```python
from build123d import *

# Parameters (mm, degrees)
SKETCH1_R               = 2.413
BOSS_EXTRUDE1_DEPTH     = 1.7859375
SKETCH6_R               = 3.956130657
SKETCH6_R_2             = 2.413
BOSS_EXTRUDE2_DEPTH     = 0.381
SKETCH5_OUTSIDE_W       = 46.08
SKETCH5_OUTSIDE_H       = 47.552
SKETCH5_OUTSIDE_R       = 4.7625
CUT_EXTRUDE2_DEPTH      = 9.104416837
CUT_EXTRUDE2_DRAFT      = -60
MIRROR1_COPY_1_SKETCH_W = 46.08
MIRROR1_COPY_1_SKETCH_H = 47.552
MIRROR1_COPY_1_SKETCH_R = 4.7625
MIRROR1_COPY_1_DEPTH    = 9.104416837
MIRROR1_COPY_1_DRAFT    = -60


with BuildPart() as part:
    # Sketch1 → Boss-Extrude1 (new, symmetric)
    with BuildSketch(Plane(origin=(0, 0, 0), x_dir=(1, 0, 0), z_dir=(0, 1, 0))):
        Polygon((-4.7625, 2.749630657), (-4.7625, -2.749630657), (0, -5.499261314), (4.7625, -2.749630657), (4.7625, 2.749630657), (0, 5.499261314), align=None)
        with Locations(Location((0, 0, 0), (0, 0, 270))):
            Circle(SKETCH1_R, mode=Mode.SUBTRACT)
    extrude(amount=BOSS_EXTRUDE1_DEPTH, both=True)

    # Sketch6 → Boss-Extrude2 (add)
    with BuildSketch(Plane(origin=(0, 1.7859375, 0), x_dir=(1, 0, 0), z_dir=(0, 1, 0))):
        with Locations(Location((0, 0, 0), (0, 0, 90))):
            Circle(SKETCH6_R)
        with Locations(Location((0, 0, 0), (0, 0, 270))):
            Circle(SKETCH6_R_2, mode=Mode.SUBTRACT)
    extrude(amount=BOSS_EXTRUDE2_DEPTH)


with BuildPart() as cut_extrude2_tool:
    # Sketch5 outside → Cut-Extrude2 (with draft: the straight prism first)
    with BuildSketch(Plane(origin=(0, 1.7859375, 0), x_dir=(1, 0, 0), z_dir=(0, 1, 0))):
        Rectangle(SKETCH5_OUTSIDE_W, SKETCH5_OUTSIDE_H)
        Circle(SKETCH5_OUTSIDE_R, mode=Mode.SUBTRACT)
    extrude(amount=-CUT_EXTRUDE2_DEPTH)
    # Cut-Extrude2: the draft: its side faces are tilted about the plane it starts from
    cut_extrude2_sides = [cut_extrude2_tool.faces().sort_by_distance(p)[0] for p in [
        (0, -2.766270918, 23.776),
        (23.04, -2.766270918, 0),
        (0, -2.766270918, -23.776),
        (-23.04, -2.766270918, 0),
        (-4.7625, -2.766270918, 0),
    ]]
    draft(cut_extrude2_sides, Plane(origin=(0, 1.7859375, 0), x_dir=(1, 0, 0), z_dir=(0, 1, 0)), CUT_EXTRUDE2_DRAFT)


with BuildPart() as part_1:
    add(part.part)

    # Cut-Extrude2: cut by cut_extrude2_tool
    add(cut_extrude2_tool.part, mode=Mode.SUBTRACT)


with BuildPart() as mirror1_copy_1_tool:
    # Mirror1 copy 1 sketch → Mirror1 copy 1 (with draft: the straight prism first)
    with BuildSketch(Plane.XZ.offset(1.7859375)):
        Rectangle(MIRROR1_COPY_1_SKETCH_W, MIRROR1_COPY_1_SKETCH_H)
        Circle(MIRROR1_COPY_1_SKETCH_R, mode=Mode.SUBTRACT)
    extrude(amount=-MIRROR1_COPY_1_DEPTH)
    # Mirror1 copy 1: the draft: its side faces are tilted about the plane it starts from
    mirror1_copy_1_sides = [mirror1_copy_1_tool.faces().sort_by_distance(p)[0] for p in [
        (0, 2.766270918, 23.776),
        (23.04, 2.766270918, 0),
        (0, 2.766270918, -23.776),
        (-23.04, 2.766270918, 0),
        (-4.7625, 2.766270918, 0),
    ]]
    draft(mirror1_copy_1_sides, Plane.XZ.offset(1.7859375), MIRROR1_COPY_1_DRAFT)


with BuildPart() as part_2:
    add(part_1.part)

    # Mirror1 copy 1: cut by mirror1_copy_1_tool
    add(mirror1_copy_1_tool.part, mode=Mode.SUBTRACT)


solid = part_2.part
```
Work out the finished part from the listing and answer in its coordinate system (mm). A direction names the side the tool comes from. Give positions to 0.01 mm unless a question says otherwise; leave off trailing zeros. Order: outer loops, then holes, each group sorted by start corner. A loop starts at its lowest first (then second) coordinate and runs counter-clockwise, first axis right, second up. Notation, with made-up numbers: (-26, 72) - (-1, 72) arc R8 cw to (-1, 84) - close; hole circle Ø5 at (-19, -39). An arc over 180 degrees is marked (long way). One line per item, written item: value. Start each with the question number.
1. Section A-A, the plane y = -0.85 is taken. Write down the section's boundary in (x, z), then the cut area to 3 significant figures.
2. Each of these flat-tipped pins is pushed along its axis until it touches: pin 1 Ø1 at (x, z) = (3.5, -4) entering from -Y; pin 2 Ø1 at (y, z) = (-1, -4) entering from -X; pin 3 Ø2 at (x, y) = (2, -0.5) entering from -Z. Where does it stop, or does it pass through?
3. For a pull along X with two mould halves and no side action, classify faces 1 (the face through (-1.468, 0.163, -1.915)), 2 (the face through (4.762, 0, 0)), 3 (the face through (2, -1.786, 2)) as released by +X, released by -X, zero draft, split by the parting line, or undercut.
4. Which of the six approach directions +Z, -Z, +X, -X, +Y, -Y give full straight-line access (tool end or side, diameter ignored) to faces 4 (the face through (3.86, 1.97, 0.86)), 5 (the face through (-4.271, 1.685, -2.48))?
5. Consider line 1 (X direction, y = -0.3, z = 0); line 2 (Y direction, x = 3.5, z = -2.5); line 3 (X direction, y = -1.3, z = -2). Determine where each line is inside the solid, lowest interval first.
Filled sheet:
1. outline: (-4.76, -2.75) - (0, -5.5) - (4.76, -2.75) - (4.76, 2.75) - (0, 5.5) - (-4.76, 2.75) - close; hole circle Ø4.83 at (0, 0)
1. area: 60.3 mm²
2. pin 1: y = -1.76
2. pin 2: x = -3.46
2. pin 3: z = -4.92
3. face 1: undercut
3. face 2: released by +X
3. face 3: zero draft
4. face 4: +Y
4. face 5: -Z, -X, +Y
5. line 1: -4.76 to -2.41, 2.41 to 4.76
5. line 2: -1.79 to 1.79
5. line 3: -4.76 to -1.35, 1.35 to 4.76
